from build123d import *

# Parameters (mm, degrees)
EXTRUDE_1_DEPTH     = 1.5
CUT_EXTRUDE_1_DEPTH = 4
FILLET_1_R          = 1
SKETCH_3_W          = 25
SKETCH_3_H          = 18.375
CUT_EXTRUDE_2_DEPTH = 4
FILLET_2_R          = 2
SKETCH_4_R          = 2.025
CUT_EXTRUDE_3_DEPTH = 10
FILLET_3_R          = 3
FILLET_4_R          = 2


with BuildPart() as part:
    # 草图1 → 凸台-拉伸1 (new body, symmetric)
    with BuildSketch(Plane.XY):
        Polygon((0, 0), (-60, 0), (-60, 20), (-40, 90), (0, 90), align=None)
    extrude(amount=EXTRUDE_1_DEPTH, both=True)

    # 草图2 → 切除-拉伸1 (cut, through all)
    with BuildSketch(Plane.XY.offset(1.5)):
        Polygon((-40, 71.799725277), (-54.799921508, 20), (-40, 20), align=None)
    extrude(amount=-CUT_EXTRUDE_1_DEPTH, mode=Mode.SUBTRACT)

    # 圆角1
    fillet_1_edges = [part.edges().sort_by_distance(p)[0] for p in [
        (-40, 71.799725277, 0),
        (-40, 20, 0),
    ]]
    fillet(fillet_1_edges, radius=FILLET_1_R)

    # 草图3 → 切除-拉伸2 (cut, through all)
    with BuildSketch(Plane.XY.offset(1.5)):
        with Locations((-20, 68.8125)):
            Rectangle(SKETCH_3_W, SKETCH_3_H)
        with Locations((-20, 38.4375)):
            Rectangle(SKETCH_3_W, SKETCH_3_H)
    extrude(amount=-CUT_EXTRUDE_2_DEPTH, mode=Mode.SUBTRACT)

    # 圆角2
    fillet_2_edges = [part.edges().sort_by_distance(p)[0] for p in [
        (-7.5, 78, 0),
        (-7.5, 59.625, 0),
        (-32.5, 59.625, 0),
        (-32.5, 78, 0),
        (-7.5, 47.625, 0),
        (-7.5, 29.25, 0),
        (-32.5, 29.25, 0),
        (-32.5, 47.625, 0),
    ]]
    fillet(fillet_2_edges, radius=FILLET_2_R)

    # 草图4 → 切除-拉伸3 (cut)
    with BuildSketch(Plane.XY.offset(1.5)):
        with Locations((-50, 10)):
            Circle(SKETCH_4_R)
        with Locations((-20, 10)):
            Circle(SKETCH_4_R)
        with Locations((-20, 24)):
            Circle(SKETCH_4_R)
        with Locations((-20, 52.5)):
            Circle(SKETCH_4_R)
        with Locations((-20, 83.5)):
            Circle(SKETCH_4_R)
    extrude(amount=-CUT_EXTRUDE_3_DEPTH, mode=Mode.SUBTRACT)

    # 圆角3
    fillet_3_edges = [part.edges().sort_by_distance(p)[0] for p in [
        (0, 0, 0),
        (-60, 0, 0),
        (-60, 20, 0),
        (-40, 90, 0),
        (0, 90, 0),
    ]]
    fillet(fillet_3_edges, radius=FILLET_3_R)

    # 圆角4
    fillet_4_edges = [part.edges().sort_by_distance(p)[0] for p in [
        (-54.799921508, 20, 0),
    ]]
    fillet(fillet_4_edges, radius=FILLET_4_R)


solid = part.part
Here's how the part is built. I have some questions about the finished solid (model axes, mm). A direction names the side the tool comes from. Round coordinates to 2 decimals unless told otherwise and drop trailing zeros. Loops run counter-clockwise (first coordinate to the right, second up) from the corner with the lowest first, then second, coordinate; pieces in that order, holes last. Notation, with made-up numbers: (74, -5.5) - (128, -5.5) arc R21 cw to (128, 32.5) - close; hole circle Ø1 at (-21.75, -1). An arc over 180 degrees is marked (long way). One line per question, with ' | ' between items. Start each with the question number.
Q1. I want a section at D-D (x = -50). Write out the boundary of the cut face in (y, z) (3 decimals), then the cut area to 3 significant figures.
Q2. I want a section at C-C (y = 83.5). Write out the boundary of the cut face in (x, z) (3 decimals).
Q3. I want a section at A-A (y = 10). Write out the boundary of the cut face in (x, z) (3 decimals).
Q4. For faces 4 (the flat face through (-47.93, 44.04, 0.02)), 5 (the flat face through (-60, 11, 0)), which set-ups out of +Z, -Z, +X, -X, +Y, -Y let a thin tool reach every point of the face, with its end or its side?
Q5. I want a section at B-B (x = -43). Write out the boundary of the cut face in (y, z), then the cut area to 3 significant figures.
Q6. Will these pins go through, and if not, where does the flat tip stop? pin 1 (4.5 mm diameter, centred on x = -20, y = 10, fed in from +Z); pin 2 (0.9 mm diameter, centred on y = 66.5, z = 0.5, fed in from -X); pin 3 (1.5 mm diameter, centred on y = 39.5, z = 0.5, fed in from -X).
Q7. Please list where these lines run through material, in increasing order: line 1 (Y direction, x = -25.5, z = -0.75) (3 decimals); line 2 (X direction, y = 44.5, z = 0.35); line 3 (X direction, y = 38, z = -0.6). Write a range as [from, to].
Q8. We'd pull the mould along X, two halves only. Please class faces 1 (the cylindrical face through (-31.899, 60.195, -0.021)), 2 (the flat face through (0, 46, 0)), 3 (the cylindrical face through (-39.522, 89.411, 0.021)): +X half, -X half, draft (parallel to the pull), parting line (faces both ways), or undercut.
Response values:
1) outline: (0, -1.5) - (7.975, -1.5) - (7.975, 1.5) - (0, 1.5) - close; (12.025, -1.5) - (20, -1.5) - (20, 1.5) - (12.025, 1.5) - close; (36.8, -1.5) - (55, -1.5) - (55, 1.5) - (36.8, 1.5) - close | area: 102 mm²
2) outline: (-41.857, -1.5) - (-22.025, -1.5) - (-22.025, 1.5) - (-41.857, 1.5) - close; (-17.975, -1.5) - (0, -1.5) - (0, 1.5) - (-17.975, 1.5) - close
3) outline: (-60, -1.5) - (-52.025, -1.5) - (-52.025, 1.5) - (-60, 1.5) - close; (-47.975, -1.5) - (-22.025, -1.5) - (-22.025, 1.5) - (-47.975, 1.5) - close; (-17.975, -1.5) - (0, -1.5) - (0, 1.5) - (-17.975, 1.5) - close
4) face 4: +Z, -Z | face 5: +Z, -Z, -X, +Y, -Y
5) outline: (0, -1.5) - (20, -1.5) - (20, 1.5) - (0, 1.5) - close; (61.3, -1.5) - (79.5, -1.5) - (79.5, 1.5) - (61.3, 1.5) - close | area: 115 mm²
6) pin 1: stops at z = 1.5 | pin 2: stops at x = -46.84 | pin 3: stops at x = -54.64
7) line 1: y = [0, 29.25], [47.625, 59.625], [78, 90] | line 2: x = [-53, -47.8], [-40, -32.5], [-7.5, 0] | line 3: x = [-54.86, -49.66], [-40, -32.5], [-7.5, 0]
8) face 1: undercut | face 2: +X half | face 3: -X half
